Input: part model. Units: mm. Frame: model coordinates. Face numbers are marked on the shaded views. A direction names the side the tool comes from. Give positions to 0.01 mm unless a question says otherwise; leave off trailing zeros. Loops run counter-clockwise (first coordinate to the right, second up) from the corner with the lowest first, then second, coordinate; pieces in that order, holes last. Notation, with made-up numbers: (79, 64) - (125, 64) arc R25 ccw to (125, 93) - close; hole circle Ø8 at (66.5, -23). An arc over 180 degrees is marked (long way). One line per item, written item: value.
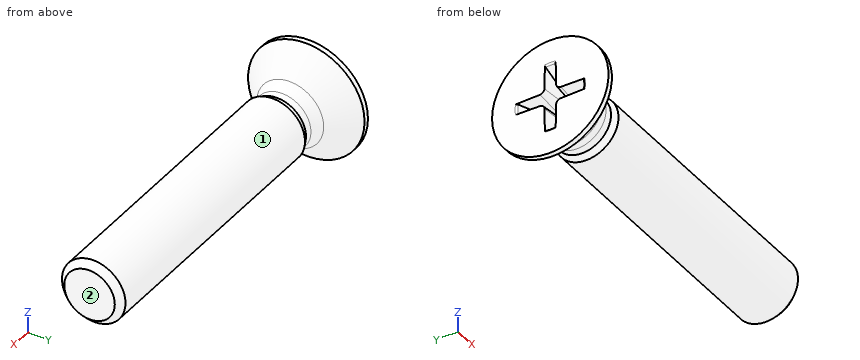
Autodesk Inventor part; units mm, degrees
ref_plane "Work Plane2" through (3.35, 0, 0) normal (0, 0, -1) x (1, 0, 0)
ref_plane "YZ Plane" through (0, 0, 0) normal (1, 0, 0) x (0, 1, 0)
ref_plane "XZ Plane" through (0, 0, 0) normal (0, 1, 0) x (-1, 0, 0)
sketch "Sketch1" plane through (0, 0, 0) normal (0, 0, 1) x (1, 0, 0)
  line L0 (2.1, 0) -> (16, 0)
  line L1 (16, 0) -> (16, 1.5)
  line L2 (16, 1.5) -> (2.65, 1.5)
  line L3 (2.65, 1.5) -> (2.3433, 1.3466)
  line L4 (2.3433, 1.3466) -> (1.9814, 1.3466)
  line L5 (0, 2.75) -> (0, 1.6)
  line L6 (0, 1.6) -> (1.6999, 0.7525)
  line L7 (1.6999, 0.7525) -> (2.1, 0)
  line L8 (-3.2, 0) -> (19.2, 0)
  line L9 (0, -0.55) -> (0, 3.3)
  line L10 (0, 2.75) -> (0.2466, 2.75)
  line L11 (0.2466, 2.75) -> (1.4157, 1.581)
  line L12 (2.65, 1.5) -> (1.4966, 1.5) construction
  arc A0 (1.4157, 1.581) -> (1.9814, 1.3466) centre (1.9814, 2.1466) ccw
  point P0 (1.65, 1.3466)
  dimension "d1" = 13.35
  dimension "d2" = 3
  dimension "d3" = 2.6933
  dimension "d4" = 3.2
  dimension "d5" = 26.5
  dimension "d6" = 62
  dimension "d7" = 2.1
  dimension "d8" = 0.3067
  dimension "d12" = 5.5
  dimension "d13" = 45
  dimension "d15" = 16
  dimension "d24" = 1.65
  dimension "d93" = 0.8
revolve "Body" add sketch "Sketch1" angle 360 about axis through (2.1, 0, 0) along (1, 0, 0) contours L7 L6 L5 L10 L11 A0 L4 L3 L2 L1 L0
sketch "Sketch2" plane through (0, 0, 0) normal (-1, 0, 0) x (0, 0, 1)
  line L0 (0, 1.6) -> (0, 0) construction
  line L1 (0, 0) -> (1.6, 0) construction
  arc A0 (0.48, 0) -> (0, 0.48) centre (0, 0) ccw construction
  arc A1 (0.56, 0) -> (0, 0.56) centre (0, 0) ccw construction
  arc A2 (1.5795, 0.255) -> (0.255, 1.5795) centre (0, 0) ccw
  line L2 (0, 0) -> (1.1314, 1.1314) construction
  line L3 (0.255, 1.5795) -> (0.2766, 0.4869)
  line L4 (1.5795, 0.255) -> (0.4869, 0.2766)
  arc A3 (0.255, 1.5795) -> (0, 1.6) centre (0, 0) ccw
  arc A4 (1.6, 0) -> (1.5795, 0.255) centre (0, 0) ccw
  line L5 (0, -3.85) -> (0, 3.85)
  line L6 (-3.85, 0) -> (3.85, 0)
  arc A5 (0.255, -1.5795) -> (1.5795, -0.255) centre (0, 0) ccw
  line L7 (0.255, -1.5795) -> (0.2766, -0.4869)
  line L8 (1.5795, -0.255) -> (0.4869, -0.2766)
  arc A6 (0, -1.6) -> (0.255, -1.5795) centre (0, 0) ccw
  arc A7 (1.5795, -0.255) -> (1.6, 0) centre (0, 0) ccw
  arc A8 (-0.255, 1.5795) -> (-1.5795, 0.255) centre (0, 0) ccw
  line L9 (-0.255, 1.5795) -> (-0.2766, 0.4869)
  line L10 (-1.5795, 0.255) -> (-0.4869, 0.2766)
  arc A9 (0, 1.6) -> (-0.255, 1.5795) centre (0, 0) ccw
  arc A10 (-1.5795, 0.255) -> (-1.6, 0) centre (0, 0) ccw
  arc A11 (-0.255, -1.5795) -> (0, -1.6) centre (0, 0) ccw
  arc A12 (-1.5795, -0.255) -> (-0.255, -1.5795) centre (0, 0) ccw
  arc A13 (-1.6, 0) -> (-1.5795, -0.255) centre (0, 0) ccw
  line L11 (-1.5795, -0.255) -> (-0.4869, -0.2766)
  line L12 (-0.255, -1.5795) -> (-0.2766, -0.4869)
  arc A14 (0.2766, 0.4869) -> (0.4869, 0.2766) centre (0.4912, 0.4912) ccw
  arc A15 (0.4869, -0.2766) -> (0.2766, -0.4869) centre (0.4912, -0.4912) ccw
  arc A16 (-0.4869, 0.2766) -> (-0.2766, 0.4869) centre (-0.4912, 0.4912) ccw
  arc A17 (-0.2766, -0.4869) -> (-0.4869, -0.2766) centre (-0.4912, -0.4912) ccw
  point P0 (1.1314, -1.1314)
  point P1 (-1.1314, 1.1314)
  point P2 (-1.1314, -1.1314)
  dimension "d17" = 0.96
  dimension "d18" = 1.12
  dimension "d19" = 3.2
  dimension "d20" = 45
  dimension "d21" = 0.255
extrude "Slot" add sketch "Sketch2" against normal up to next draft 5 contours L4 A14 L3 A2 | A5 L7 A15 L8 | L9 A16 L10 A8 | A12 L11 A17 L12
fillet "Fillet1" radius 0.102 4 edges at (0, 1.6, 0) (0, 0, -1.6) (0, -1.6, 0) (0, 0, 1.6)
thread "Thread"
chamfer "Chamfer1" distance 0.3067 distance2 0.3069 1 edges at (16, -1.5, 0) measured on face at (16, -0.5495, 0.6466)
ref_plane "Work Plane2" through (3.35, 0, 0) normal (0, 0, -1) x (1, 0, 0)
equation "\"d17\" = 0.3 * SDM"
equation "\"d18\" = 0.35 * SDM"
equation "\"d19\" = SDM"
equation "\"d21\" = 0.5 * SBR"
equation "\"d1\" = GEL"
equation "\"d2\" = GD"
equation "\"d3\" = BDM"
equation "\"d4\" = SDM"
equation "\"d7\" = INTI"
equation "\"d8\" = GAL"
equation "\"d12\" = KOD"
equation "\"d13\" = 0.5 * SEWI"
equation "\"d15\" = NLG"
equation "\"d93\" = R"
equation "\"d23\" = 0.2 * SBR"
equation "\"d10\" = GEL"
equation "\"d25\" = -0.5 * SPD + 0.5 * GD"
equation "\"NLG\" = 16"
equation "\"GEL\" = 13.35"
equation "\"GAL\" = 0.61345 * PTC"
equation "\"SPD\" = NND - 1.2269 * PTC"
equation "\"KOD\" = 5.5"
equation "\"KOH\" = 1.65"
equation "\"SBR\" = 0.51"
equation "\"INTI\" = 2.1"
equation "\"SDM\" = 3.2"
equation "\"GD\" = NND"
equation "\"BDM\" = NND - GAL"
equation "\"SEWI\" = 90deg"
equation "\"d9\" = SDM"
equation "\"R\" = 0.8"
equation "\"GUL\" = 0.61345 * PTC"
equation "\"TOA\" = 30deg"
equation "\"EPV\" = 3.15"
equation "\"THREADDIA\" = 3"
equation "\"PTC\" = 0.5"
equation "\"NND\" = 3"
equation "\"GD1\" = THREADDIA - 1.2269 * PTC"
properties part number "ISO 7046-1  - M3 x 16 - 4.8 - H" material "Steel"
Item 1: Section A-A, the plane x = 5. Output: boundary loops of the cut face in (y, z).
Verdict:
outline: circle Ø3 at (0, 0)
Item 2: Pin query (flat end, axial travel): P1, Ø1, axis at y = 1, z = 0.5, coming from the -X side; P2, Ø1, axis at x = 7, y = 0.5, coming from the +Z side. Return the tip coordinate at first contact, or that it passes through.
Verdict:
P1: stops at x = 0
P2: stops at z = 1.5
Item 3: Material intervals for L1, parallel to X at y = -1.6, z = -0.4; L2, parallel to Z at x = 4.5, y = -1.3; L3, parallel to X at y = -0.3, z = -1.6, sorted ascending.
Verdict:
L1: x = 0 to 1.35
L2: z = -0.75 to 0.75
L3: x = 0 to 1.37
Item 4: Access query for the marked faces 1 and 2. Directions: +Z, -Z, +X, -X, +Y, -Y. A direction counts if a zero-diameter tool reaches every point of the face in a straight line with its end or side. Return the directions, or none.
Verdict:
face 1: +X
face 2: +Z, -Z, +X, +Y, -Y
